from build123d import *

# Parameters (mm, degrees)
F0_W     = 44
F0_H     = 11
F1_DEPTH = 11.9
F2_R     = 6.25
F3_DEPTH = 25
F4_R     = 8.25
F5_DEPTH = 5
F6_R     = 8.75
F7_DEPTH = 2.8
F8_R     = 1.6
F8_R_2   = 11.25
F9_DEPTH = 25
F11_R    = 2.25


with BuildPart() as f1:
    # F0 (on Top) → F1 (new body)
    with BuildSketch(Plane.XY):
        with Locations((22, 5.5)):
            Rectangle(F0_W, F0_H)
    extrude(amount=F1_DEPTH)

    # F2 (on face) → F3 (cut)
    with BuildSketch(Plane.XY.offset(11.9)):
        with Locations((29, 11)):
            Circle(F2_R)
    extrude(amount=-F3_DEPTH, mode=Mode.SUBTRACT)

    # F4 (on face) → F5 (cut)
    with BuildSketch(Plane.XY.offset(11.9)):
        with Locations((29, 11)):
            Circle(F4_R)
    extrude(amount=-F5_DEPTH, mode=Mode.SUBTRACT)

    # F6 (on face) → F7 (cut)
    with BuildSketch(Plane(origin=(0, 0, 0), x_dir=(1, 0, 0), z_dir=(0, 0, -1))):
        with Locations((29, -11)):
            Circle(F6_R)
    extrude(amount=-F7_DEPTH, mode=Mode.SUBTRACT)

    # F8 (on face) → F9 (cut)
    with BuildSketch(Plane.XZ):
        with Locations((39.440233, 5.15)):
            Circle(F8_R)
        with Locations((7.940233, 5.15)):
            Circle(F8_R)
        with Locations((23.690233, 20.9)):
            Circle(F8_R_2)
    extrude(amount=-F9_DEPTH, mode=Mode.SUBTRACT)

    # F12: sweep along a path in F10
    with BuildLine(Plane(origin=(0, 11, 0), x_dir=(-1, 0, 0), z_dir=(0, 1, 0))) as f12_path:
        Line((-22.5, -6.5), (-2.5, 16.9))
    # F11 (on face) → F12 (sweep, cut)
    with BuildSketch(Plane(origin=(0, 0, 0), x_dir=(1, 0, 0), z_dir=(0, 0, -1))):
        with Locations((19.15, -11)):
            Circle(F11_R)
    sweep(path=f12_path.line, mode=Mode.SUBTRACT)


solid = f1.part
Verification items for the finished model (mm, model axes). A direction names the side the tool comes from. Give positions to 0.01 mm unless a question says otherwise; leave off trailing zeros. Order: outer loops, then holes, each group sorted by start corner. A loop starts at its lowest first (then second) coordinate and runs counter-clockwise, first axis right, second up. Notation, with made-up numbers: M 73,27.25 L 94,27.25 A20 cw 94,40.25 Z; hole C -5.5,39 d1. An arc over 180 degrees is marked long. Answer as a JSON object with one key per item and string values. Group by question number.
1) Cross-section at C-C (x = 29). Enter the section's corners in (y, z).
2) Mould release check, pull along Z, two halves, no side actions. Record for faces 1 (the face through (40.966, 5.423, 5.631)), 2 (the face through (6.76, 5.42, 6.23)), 3 (the face through (0, 5, 6)), 4 (the face through (39, 4, 11.9)): released by +Z, released by -Z, zero draft, split by the parting line, or undercut.
3) Access from +Z, -Z, +X, -X, +Y, -Y to the whole of each face (thin tool, end or side, straight path). Record for faces 5 (the face through (29.192, 2.252, 1.38)), 6 (the face through (6, 11, 5)), 7 (the face through (28, 4, 6.9)).
4) Cross-section at D-D (z = 5.15). Give the number of separate pieces and of enclosed holes in the cut face, then the cut area to 3 significant figures.
5) Cross-section at B-B (x = 40). Enter the section's corners in (y, z).
6) Cross-section at A-A (y = 1). Enter the section's corners in (x, z).
7) Scan lines: line 1 along X through (y, z) = (9.25, 10.75); line 2 along X through (y, z) = (9.75, 9); line 3 along X through (y, z) = (6.75, 6). Record each from-to range of solid material in increasing order. Write a range as [from, to].
Result sheet:
{
 "1": {"outline": "M 0,0 L 2.25,0 L 2.25,2.8 L 4.75,2.8 L 4.75,6.9 L 2.75,6.9 L 2.75,10.98 L 0,10.98 Z"},
 "2": {"face 1": "undercut", "face 2": "undercut", "face 3": "zero draft", "face 4": "released by +Z"},
 "3": {"face 5": "-Z, +Y", "face 6": "+Z, -Z, +X, -X, +Y", "face 7": "+Z, +Y"},
 "4": {"separate pieces": "3", "enclosed holes": "0", "area": "344 mm2"},
 "5": {"outline": "M 0,0 L 11,0 L 11,3.65 L 0,3.65 Z; M 0,6.65 L 11,6.65 L 11,11.9 L 0,11.9 Z"},
 "6": {"outline": "M 0,0 L 44,0 L 44,11.9 L 30.44,11.9 A11.25 cw 16.94,11.9 L 0,11.9 Z; hole C 7.94,5.15 d3.2; hole C 39.44,5.15 d3.2"},
 "7": {"line 1": "x = [0, 8.55], [11.38, 18.84], [37.06, 44]", "line 2": "x = [0, 9.59], [13.33, 20.85], [37.15, 44]", "line 3": "x = [0, 6.58], [9.3, 24.42], [33.58, 38.08], [40.8, 44]"}
}
